from build123d import *

# Parameters (mm, degrees)
EXTRUDE_1_DEPTH = 4
FILLET_1_R      = 3
FILLET_2_R      = 6


with BuildPart() as part:
    # ｽｹｯﾁ1 → ﾎﾞｽ - 押し出し1 (new body)
    with BuildSketch(Plane.XY):
        with BuildLine():
            Line((0, 2.5), (0, 5.5))
            Line((0, 5.5), (-7, 4.1))
            Line((-7, 4.1), (-7, -7.4))
            Line((-7, -7.4), (0, -16))
            Line((0, -16), (0, -2.5))
            ThreePointArc((0, -2.5), (-2.5, 0), (0, 2.5))
        make_face()
    extrude(amount=EXTRUDE_1_DEPTH)

    # ﾌｨﾚｯﾄ1
    fillet_1_edges = [part.edges().sort_by_distance(p)[0] for p in [
        (-7, 4.1, 2),
    ]]
    fillet(fillet_1_edges, radius=FILLET_1_R)

    # ﾌｨﾚｯﾄ2
    fillet_2_edges = [part.edges().sort_by_distance(p)[0] for p in [
        (-7, -7.4, 2),
    ]]
    fillet(fillet_2_edges, radius=FILLET_2_R)


solid = part.part
Verification items for the finished model (mm, model axes). Round coordinates to 2 decimals unless told otherwise and drop trailing zeros. Order: outer loops, then holes, each group sorted by start corner. A loop starts at its lowest first (then second) coordinate and runs counter-clockwise, first axis right, second up.
1. Go/stop test with a flat-tipped pin: P1, Ø1.5, axis at x = -2, z = 1, coming from the +Y side. Record where the tip stops, or that it passes through.
Final values:
P1: stops at y = 5.25
2. Release check for a two-part mould opening along Y. For faces 1 (the flat face through (-4, -3, 0)), 2 (the cylindrical face through (-6.663, -7.25, 2.028)), 3 (the cylindrical face through (-2.5, -0.1, 2)), 4 (the cylindrical face through (-6.302, 3.565, 2.028)) record: +Y half, -Y half, draft (parallel to the pull), parting line (faces both ways), or undercut.
Final values:
face 1: draft
face 2: -Y half
face 3: undercut
face 4: +Y half
3. Section check B-B on z = 0.4. Record the cut outline in (x, y), then the cut area to 3 significant figures.
Final values:
outline: (-7, -5.27) arc R6 ccw to (-5.65, -9.05) - (0, -16) - (0, -2.5) arc R2.5 cw to (0, 2.5) - (0, 5.5) - (-4.59, 4.58) arc R3 ccw to (-7, 1.64) - close
area: 104 mm2
4. Thickness scan on L1, parallel to Y at x = -0.25, z = 2.45; L2, parallel to Y at x = -1, z = 0.25; L3, parallel to X at y = -5.5, z = 0.2. Record the ranges inside material, lowest first.
Final values:
L1: y = -15.69 to -2.49, 2.49 to 5.45
L2: y = -14.77 to -2.29, 2.29 to 5.3
L3: x = -7 to 0
5. Section check C-C on y = 0. Record the cut outline in (x, z), then the cut area to 3 significant figures.
Final values:
outline: (-7, 0) - (-2.5, 0) - (-2.5, 4) - (-7, 4) - close
area: 18.0 mm2
6. Section check D-D on x = -5.25. Record the cut outline in (y, z), then the cut area to 3 significant figures.
Final values:
outline: (-9.55, 0) - (4.37, 0) - (4.37, 4) - (-9.55, 4) - close
area: 55.7 mm2
7. Section check A-A on x = -2. Record the cut outline in (y, z).
Final values:
outline: (-13.54, 0) - (-1.5, 0) - (-1.5, 4) - (-13.54, 4) - close; (1.5, 0) - (5.1, 0) - (5.1, 4) - (1.5, 4) - close
